Geometry: final body of the model. Coordinates: model frame, mm. Face numbers are marked on the shaded views. A direction names the side the tool comes from. Round coordinates to 2 decimals unless told otherwise and drop trailing zeros. Loops run counter-clockwise (first coordinate to the right, second up) from the corner with the lowest first, then second, coordinate; pieces in that order, holes last. Notation, with made-up numbers: M -3.5,30 L 31.5,30 A8 ccw 31.5,35 Z; hole C 17.5,-7 d9. An arc over 180 degrees is marked long. Answer as a JSON object with one key per item and string values.
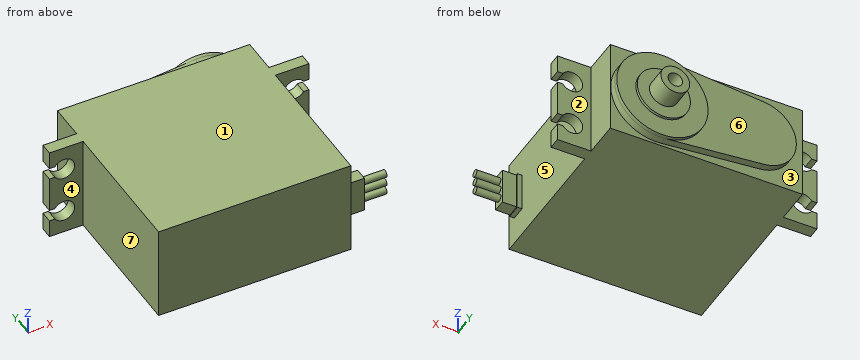
from build123d import *

# Parameters (mm, degrees)
SKETCH_1_W          = 40
SKETCH_1_H          = 20
EXTRUDE_1_DEPTH     = 29.3
EXTRUDE_2_DEPTH     = 2.5
SKETCH_3_W          = 40
SKETCH_3_H          = 20
EXTRUDE_3_DEPTH     = 7.45
EXTRUDE_4_DEPTH     = 1.53
SKETCH_5_R          = 9.5
EXTRUDE_5_DEPTH     = 0.8
SKETCH_6_R          = 3
EXTRUDE_6_DEPTH     = 5
SKETCH_7_W          = 8
SKETCH_7_H          = 3
EXTRUDE_7_DEPTH     = 1
SKETCH_8_W          = 7.6
SKETCH_8_H          = 2.6
EXTRUDE_8_DEPTH     = 3
SKETCH_9_R          = 0.75
EXTRUDE_9_DEPTH     = 5
SKETCH_10_R         = 1.5
CUT_EXTRUDE_1_DEPTH = 3
SKETCH_11_R         = 5.525
EXTRUDE_11_DEPTH    = 0.55


with BuildPart() as part:
    # 스케치1 → 보스-돌출1 (new body)
    with BuildSketch(Plane(origin=(0, 0, 0), x_dir=(1, 0, 0), z_dir=(0, 1, 0))):
        Rectangle(SKETCH_1_W, SKETCH_1_H)
    extrude(amount=EXTRUDE_1_DEPTH)

    # 스케치2 → 보스-돌출2 (add)
    with BuildSketch(Plane(origin=(0, 29.3, 0), x_dir=(1, 0, 0), z_dir=(0, 1, 0))):
        with BuildLine():
            Line((-27, 10), (27, 10))
            Line((27, 10), (27, 6.25))
            Line((27, 6.25), (25.868643032, 6.25))
            ThreePointArc((25.868643032, 6.25), (21.751817004, 5), (25.868643032, 3.75))
            Line((25.868643032, 3.75), (27, 3.75))
            Line((27, 3.75), (27, -3.75))
            Line((27, -3.75), (25.866173833, -3.75))
            ThreePointArc((25.866173833, -3.75), (21.753868932, -5), (25.866173833, -6.25))
            Line((25.866173833, -6.25), (27, -6.25))
            Line((27, -6.25), (27, -10))
            Line((27, -10), (-27, -10))
            Line((-27, -10), (-27, -6.25))
            Line((-27, -6.25), (-25.870828693, -6.25))
            ThreePointArc((-25.870828693, -6.25), (-21.75, -5), (-25.870828693, -3.75))
            Line((-25.870828693, -3.75), (-27, -3.75))
            Line((-27, -3.75), (-27, 3.75))
            Line((-27, 3.75), (-25.870828693, 3.75))
            ThreePointArc((-25.870828693, 3.75), (-21.75, 5), (-25.870828693, 6.25))
            Line((-25.870828693, 6.25), (-27, 6.25))
            Line((-27, 6.25), (-27, 10))
        make_face()
    extrude(amount=EXTRUDE_2_DEPTH)

    # 스케치3 → 보스-돌출3 (add)
    with BuildSketch(Plane(origin=(0, 31.8, 0), x_dir=(1, 0, 0), z_dir=(0, 1, 0))):
        Rectangle(SKETCH_3_W, SKETCH_3_H)
    extrude(amount=EXTRUDE_3_DEPTH)

    # 스케치4 → 보스-돌출4 (add)
    with BuildSketch(Plane(origin=(0, 39.25, 0), x_dir=(1, 0, 0), z_dir=(0, 1, 0))):
        with BuildLine():
            Line((-11.105930899, 7.466746492), (9.486550883, 9.4559828))
            ThreePointArc((9.486550883, 9.4559828), (19.9, -1.9624e-05), (9.486511816, -9.455979026))
            Line((9.486511816, -9.455979026), (-11.105960469, -7.466657767))
            ThreePointArc((-11.105960469, -7.466657767), (-17.9, 5.7816e-05), (-11.105930899, 7.466746492))
        make_face()
    extrude(amount=EXTRUDE_4_DEPTH)

    # 스케치5 → 보스-돌출5 (add)
    with BuildSketch(Plane(origin=(0, 40.78, 0), x_dir=(1, 0, 0), z_dir=(0, 1, 0))):
        with Locations(Location((10.4, 0, 0), (0, 0, 95.517659112))):
            Circle(SKETCH_5_R)
    extrude(amount=EXTRUDE_5_DEPTH)

    # 스케치6 → 보스-돌출6 (add)
    with BuildSketch(Plane(origin=(0, 41.58, 0), x_dir=(1, 0, 0), z_dir=(0, 1, 0))):
        with Locations(Location((10.4, 0, 0), (0, 0, 270))):
            Circle(SKETCH_6_R)
    extrude(amount=EXTRUDE_6_DEPTH)

    # 스케치7 → 보스-돌출7 (add)
    with BuildSketch(Plane(origin=(20, 0, 0), x_dir=(0, 0, -1), z_dir=(1, 0, 0))):
        with Locations((0, 3.5)):
            Rectangle(SKETCH_7_W, SKETCH_7_H)
    extrude(amount=EXTRUDE_7_DEPTH)

    # 스케치8 → 보스-돌출8 (add)
    with BuildSketch(Plane(origin=(21, 0, 0), x_dir=(0, 0, -1), z_dir=(1, 0, 0))):
        with Locations((0, 3.5)):
            Rectangle(SKETCH_8_W, SKETCH_8_H)
    extrude(amount=EXTRUDE_8_DEPTH)

    # 스케치9 → 보스-돌출9 (add)
    with BuildSketch(Plane(origin=(24, 0, 0), x_dir=(0, 0, -1), z_dir=(1, 0, 0))):
        with Locations((0, 3.505070748)):
            Circle(SKETCH_9_R)
        with Locations((-1.999991967, 3.499402084)):
            Circle(SKETCH_9_R)
        with Locations((1.99999474, 3.500483844)):
            Circle(SKETCH_9_R)
    extrude(amount=EXTRUDE_9_DEPTH)

    # 스케치10 → 컷-돌출1 (cut)
    with BuildSketch(Plane(origin=(0, 46.58, 0), x_dir=(1, 0, 0), z_dir=(0, 1, 0))):
        with Locations(Location((10.4, 0, 0), (0, 0, 270))):
            Circle(SKETCH_10_R)
    extrude(amount=-CUT_EXTRUDE_1_DEPTH, mode=Mode.SUBTRACT)

    # 스케치11 → 보스-돌출11 (add)
    with BuildSketch(Plane(origin=(0, 41.58, 0), x_dir=(1, 0, 0), z_dir=(0, 1, 0))):
        with Locations(Location((10.4, 0, 0), (0, 0, 270))):
            Circle(SKETCH_11_R)
    extrude(amount=EXTRUDE_11_DEPTH)


solid = part.part
1) Pin query (flat end, axial travel): P1, Ø1.3, axis at x = 22, y = 3.5, coming from the -Z side; P2, Ø1.5, axis at x = 22.5, z = -1.5, coming from the -Y side; P3, Ø7.5, axis at x = 22, z = 1, coming from the +Y side. Return the tip coordinate at first contact, or that it passes through.
Results:
{"P1": "z = -3.8", "P2": "y = 2.2", "P3": "y = 41.58"}
2) Section query C-C (y = 15). Return the cut outline in (x, z).
Results:
{"outline": "M -20,-10 L 20,-10 L 20,10 L -20,10 Z"}
3) Pull-direction query (Y, two-part tool) for the marked faces 4, 5, 6 and 7; classes: +Y half, -Y half, draft (parallel to the pull), parting line (faces both ways), or undercut.
Results:
{"face 4": "-Y half", "face 5": "undercut", "face 6": "+Y half", "face 7": "draft"}
4) Section query A-A (x = -24). Return the cut outline in (y, z), and give its area (3 significant figures).
Results:
{"outline": "M 29.3,-10 L 31.8,-10 L 31.8,-7.25 L 29.3,-7.25 Z; M 29.3,-2.75 L 31.8,-2.75 L 31.8,2.75 L 29.3,2.75 Z; M 29.3,7.25 L 31.8,7.25 L 31.8,10 L 29.3,10 Z", "area": "27.5 mm2"}
5) Section query D-D (x = -10). Return the cut outline in (y, z).
Results:
{"outline": "M 0,-10 L 39.25,-10 L 39.25,-7.57 L 40.78,-7.57 L 40.78,7.57 L 39.25,7.57 L 39.25,10 L 0,10 Z"}
6) Reachability of the marked faces 1, 2 and 3 from +Z, -Z, +X, -X, +Y, -Y: full face, straight path, thin tool, end or side. Return the list, or none.
Results:
{"face 1": "+Z, +X, -X, +Y, -Y", "face 2": "+Z, -Z, +X, +Y", "face 3": "+Y"}
7) Ray query, line 1 (Z direction, x = 24, y = 30); line 2 (X direction, y = 44.2, z = 0); line 3 (Y direction, x = 24.5, z = 0). Return the intervals inside material, ascending.
Results:
{"line 1": "-10 to -7.25, -2.75 to 2.75, 7.25 to 10", "line 2": "7.4 to 8.9, 11.9 to 13.4", "line 3": "2.76 to 4.26, 29.3 to 31.8"}
8) Section query B-B (x = 10.4). Return the cut outline in (y, z) (3 decimals), and give its area (3 significant figures).
Results:
{"outline": "M 0,-10 L 39.25,-10 L 39.25,-9.5 L 41.58,-9.5 L 41.58,-5.525 L 42.13,-5.525 L 42.13,-3 L 46.58,-3 L 46.58,-1.5 L 43.58,-1.5 L 43.58,1.5 L 46.58,1.5 L 46.58,3 L 42.13,3 L 42.13,5.525 L 41.58,5.525 L 41.58,9.5 L 39.25,9.5 L 39.25,10 L 0,10 Z", "area": "853 mm2"}
